For this review, use the dimensioned drawing (mm, ordinates from the lowest corner) and the shaded views. A direction names the side the tool comes from. Give positions to 0.01 mm unless a question says otherwise; leave off trailing zeros. Order: outer loops, then holes, each group sorted by start corner. A loop starts at its lowest first (then second) coordinate and runs counter-clockwise, first axis right, second up. Notation, with made-up numbers: (3, -18.5) - (26, -18.5) arc R32 ccw to (26, 20.5) - close; hole circle Ø5 at (20, 78). An arc over 180 degrees is marked (long way). One line per item, written item: value.
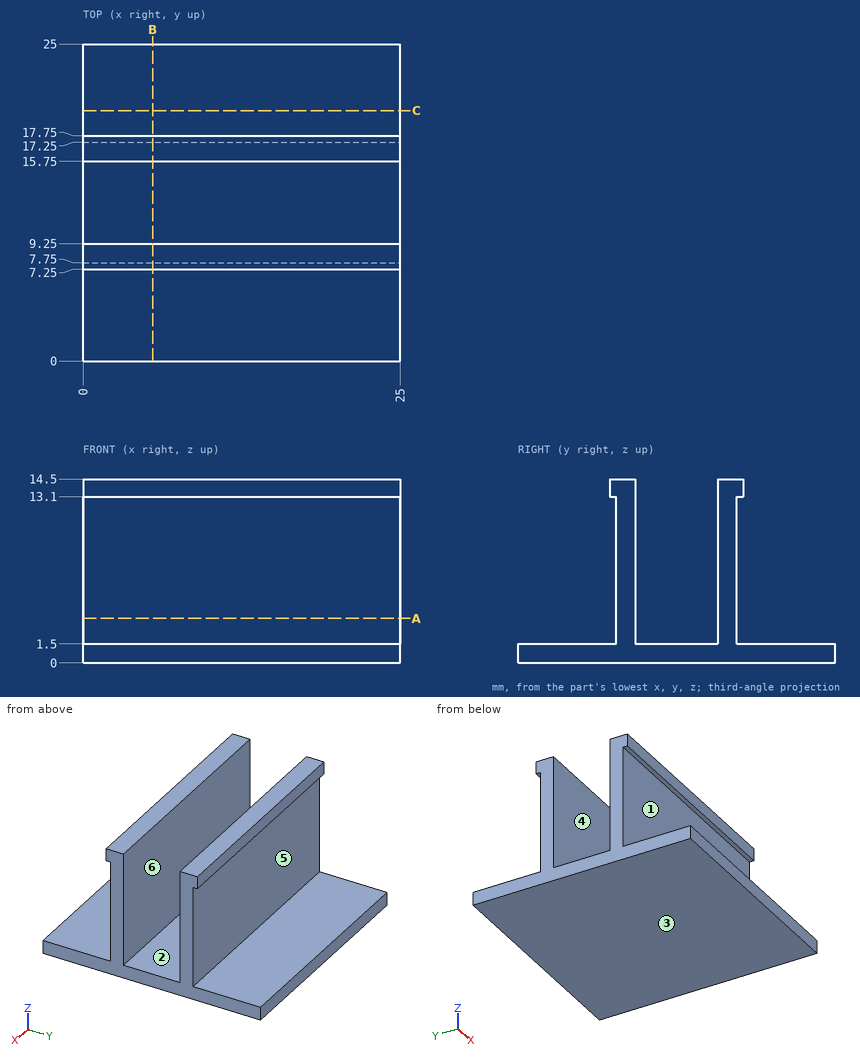
(1) Wall thickness on line 1 (Y direction, x = 3.75, z = 7.75); line 2 (Y direction, x = 10.5, z = 13.5); line 3 (Z direction, x = 15.75, y = 4.25): over which ranges is each line inside the solid? List them lowest first. Write a range as from..to.
Answers below:
line 1: y = 7.75..9.25, 15.75..17.25
line 2: y = 7.25..9.25, 15.75..17.75
line 3: z = 0..1.5
(2) Draft analysis for pull direction Y (two halves, no side actions). For the marked faces 1, 2, 3 and 4, state which applies: pulls with the +Y half, pulls with the -Y half, needs draft (parallel to the pull), parting line crosses it, or undercut.
Answers below:
face 1: pulls with the -Y half
face 2: undercut
face 3: needs draft
face 4: undercut
(3) Take a section at A-A (z = 3.5). Write out the cut boundary in (x, y).
Answers below:
outline: (0, 7.75) - (25, 7.75) - (25, 9.25) - (0, 9.25) - close; (0, 15.75) - (25, 15.75) - (25, 17.25) - (0, 17.25) - close
(4) Take a section at B-B (x = 5.5). Write out the cut boundary in (y, z).
Answers below:
outline: (0, 0) - (25, 0) - (25, 1.5) - (17.25, 1.5) - (17.25, 13.1) - (17.75, 13.1) - (17.75, 14.5) - (15.75, 14.5) - (15.75, 1.5) - (9.25, 1.5) - (9.25, 14.5) - (7.25, 14.5) - (7.25, 13.1) - (7.75, 13.1) - (7.75, 1.5) - (0, 1.5) - close
(5) Machinability: for the marked faces 5 and 6, which of the approach directions +Z, -Z, +X, -X, +Y, -Y give a long, thin tool a straight path to every point of the face, cutting with its end or side? Answer none if there is none.
Answers below:
face 5: +X, -X, +Y
face 6: +Z, +X, -X
(6) For P1, Ø4, axis at x = 4, y = 9.5, coming from the +Z side; P2, Ø1, axis at y = 6.5, z = 13, coming from the +X side; P3, Ø1.5, axis at x = 10.5, z = 14, coming from the -Y side; P4, Ø6.5, axis at x = 16, z = 6, coming from the -Y side, all flat-tipped, find the tip position at first contact; note any pin that passes through.
Answers below:
P1: stops at z = 14.5
P2: passes through
P3: stops at y = 7.25
P4: stops at y = 7.75
(7) Take a section at C-C (y = 19.75). Write out the cut boundary in (x, z).
Answers below:
outline: (0, 0) - (25, 0) - (25, 1.5) - (0, 1.5) - close
